For this review, use the dimensioned drawing (mm, ordinates from the lowest corner) and the shaded views. A direction names the side the tool comes from. Coordinates: 2 decimals unless noted, no trailing zeros. Order: outer loops, then holes, each group sorted by start corner. A loop starts at its lowest first (then second) coordinate and runs counter-clockwise, first axis right, second up. Notation, with made-up numbers: M 71,7 L 85,7 A19 cw 85,12 Z; hole C 84,5 d4. An arc over 180 degrees is marked long. One line per item, written item: value.
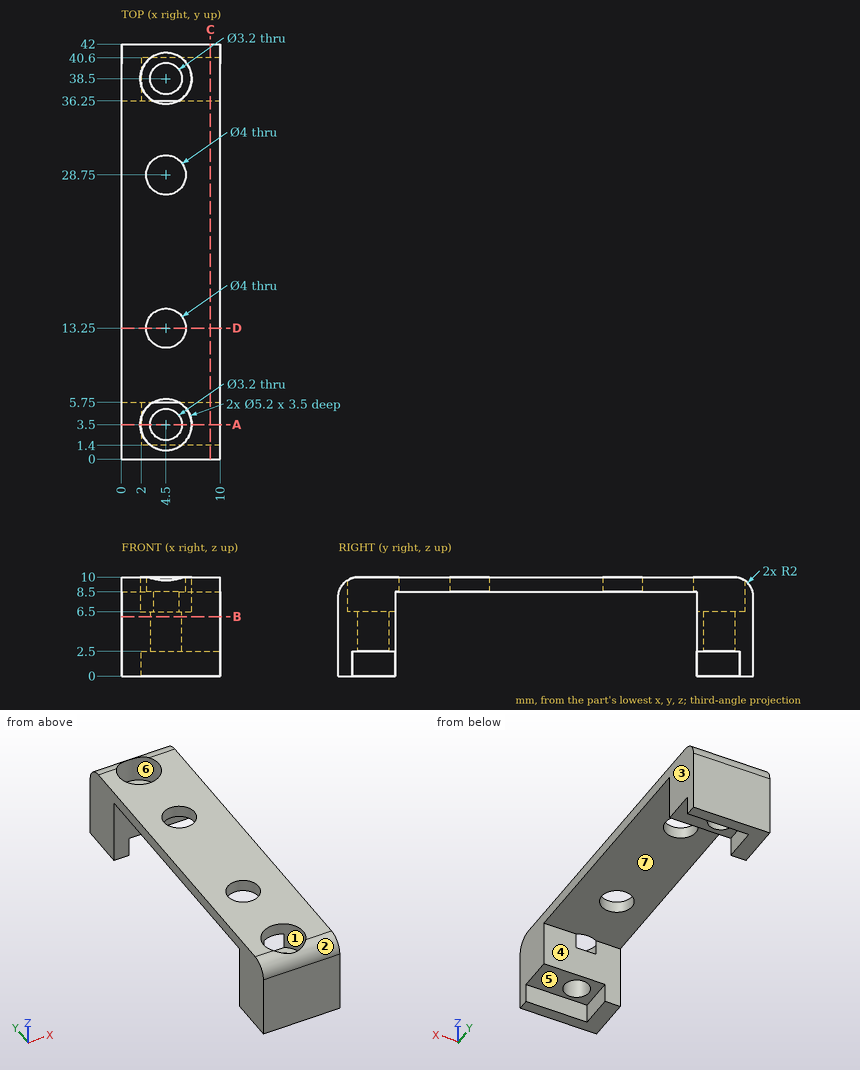
(1) We need section A-A, the plane y = 3.5. State the section outline as (x, z) points, plus the area to 3 significant figures.
Geometry results:
outline: M 0,0 L 2,0 L 2,2.5 L 2.9,2.5 L 2.9,6.5 L 1.9,6.5 L 1.9,10 L 0,10 Z; M 6.1,2.5 L 10,2.5 L 10,10 L 7.1,10 L 7.1,6.5 L 6.1,6.5 Z
area: 49.0 mm2
(2) We need section B-B, the plane z = 6. State the section outline as (x, y) points.
Geometry results:
outline: M 0,0 L 10,0 L 10,5.75 L 0,5.75 Z; M 0,36.25 L 10,36.25 L 10,42 L 0,42 Z; hole C 4.5,3.5 d3.2; hole C 4.5,38.5 d3.2
(3) Mouldability with a two-part tool opening along Y and no side actions: class the marked faces 1, 2, 3 and 4 as +Y half, -Y half, draft (parallel to the pull), parting line (faces both ways), or undercut.
Geometry results:
face 1: undercut
face 2: -Y half
face 3: draft
face 4: undercut
(4) For L1, parallel to Y at x = 4.5, z = 4.9; L2, parallel to Y at x = 8.5, z = 3.5; L3, parallel to Y at x = 4.5, z = 7.95, list the stretches that pass through material, from the lowest coordinate up.
Geometry results:
L1: y = 0 to 1.9, 5.1 to 5.75, 36.25 to 36.9, 40.1 to 42
L2: y = 0 to 5.75, 36.25 to 42
L3: y = 0 to 0.9, 41.1 to 42
(5) Insertion check: pin 1 Ø2.5 at (x, y) = (4.5, 39) entering from +Z; pin 2 Ø1 at (x, y) = (3, 23.5) entering from -Z; pin 3 Ø1.9 at (x, y) = (4.5, 38.5) entering from +Z; pin 4 Ø0.8 at (y, z) = (37.5, 1) entering from +X. Each pin has a flat end and moves straight along its axis. Give the tip position at first contact, or say it passes through.
Geometry results:
pin 1: stops at z = 6.5
pin 2: stops at z = 8.5
pin 3: passes through
pin 4: stops at x = 2
(6) We need section D-D, the plane y = 13.25. State the section outline as (x, z) points, plus the area to 3 significant figures.
Geometry results:
outline: M 0,8.5 L 2.5,8.5 L 2.5,10 L 0,10 Z; M 6.5,8.5 L 10,8.5 L 10,10 L 6.5,10 Z
area: 9.00 mm2
(7) We need section C-C, the plane x = 9. State the section outline as (y, z) points.
Geometry results:
outline: M 0,0 L 1.4,0 L 1.4,2.5 L 5.75,2.5 L 5.75,8.5 L 36.25,8.5 L 36.25,2.5 L 40.6,2.5 L 40.6,0 L 42,0 L 42,8 A2 ccw 40,10 L 2,10 A2 ccw 0,8 Z
(8) Tool access review of the marked faces 5, 6 and 7: name each direction out of +Z, -Z, +X, -X, +Y, -Y from which nothing blocks a thin tool from reaching the whole face with its end or side.
Geometry results:
face 5: -Z, +X
face 6: +Z
face 7: -Z, +X, -X
